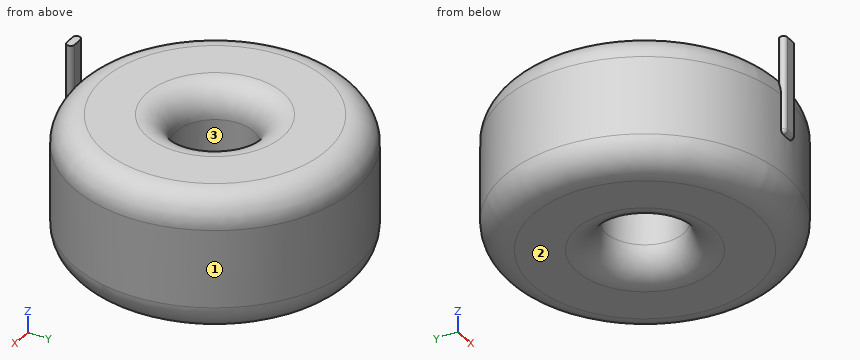
```python
from build123d import *

# Parameters (mm, degrees)
F0_R     = 72.5
F0_R_2   = 20
F1_DEPTH = 35
F2_R     = 15
F4_DEPTH = 50
F5_R     = 1.9999


# Not quite as in the source:
# - a fillet or chamfer is up to 0.001 mm smaller than in the source, because OpenCascade refuses the exact size


with BuildPart() as f1:
    # F0 (on Top) → F1 (new body, symmetric)
    with BuildSketch(Plane.XY):
        Circle(F0_R)
        Circle(F0_R_2, mode=Mode.SUBTRACT)
    extrude(amount=F1_DEPTH, both=True)

    # F2
    f2_edges = [f1.edges().sort_by_distance(p)[0] for p in [
        (-20, 0, 35),
        (20, 0, 0),
        (-20, 0, -35),
        (-72.5, 0, -35),
        (72.5, 0, 0),
        (-72.5, 0, 35),
    ]]
    fillet(f2_edges, radius=F2_R)

    # F3 (on Top) → F4 (join)
    with BuildSketch(Plane.XY):
        with BuildLine():
            Line((2.5, -70.4568837309), (-2.5, -70.4568837309))
            ThreePointArc((-2.5, -70.4568837309), (-4.5, -72.4568837309), (-2.5, -74.4568837309))
            Line((-2.5, -74.4568837309), (2.5, -74.4568837309))
            ThreePointArc((2.5, -74.4568837309), (4.5, -72.4568837309), (2.5, -70.4568837309))
        make_face()
    extrude(amount=F4_DEPTH)

    # F5 (radius 2 in the source; OpenCascade refuses exactly that, so slightly less here)
    f5_edges = [f1.edges().sort_by_distance(p)[0] for p in [
        (0, -74.456884, 0),
    ]]
    fillet(f5_edges, radius=F5_R)


solid = f1.part
```
Design review of the part built by this model. Coordinates are the model's own, in mm. Face numbers are marked on the shaded views. Give positions to 0.01 mm unless a question says otherwise; leave off trailing zeros. Loops run counter-clockwise (first coordinate to the right, second up) from the corner with the lowest first, then second, coordinate; pieces in that order, holes last. Notation, with made-up numbers: M 64,28.5 L 74,28.5 A21 ccw 74,67.5 Z; hole C 10.25,83.25 d8. An arc over 180 degrees is marked long. Return JSON: item names as keys, results as strings. Group by question number.
Item 1: For probe 1 along Y at (x, z) = (0, 9); probe 2 along Y at (x, z) = (0, -10); probe 3 along Z at (x, y) = (23, 53), list the stretches that pass through material, from the lowest coordinate up.
Item 2: We need section A-A (y = 0). Give the boundary of the cut face in (x, z).
Item 3: We need section C-C (z = -4). Give the boundary of the cut face in (x, y), and give its area (3 significant figures).
Item 4: We need section D-D (z = 7.5). Give the boundary of the cut face in (x, y), and give its area (3 significant figures).
Item 5: Insertion check: pin 1 Ø1.5 at (y, z) = (30.5, 28) entering from -X; pin 2 Ø1 at (y, z) = (30.5, -10.5) entering from -X; pin 3 Ø1 at (x, y) = (-54.5, 28.5) entering from +Z. Each pin has a flat end and moves straight along its axis. Give the tip position at first contact, or say it passes through.
Item 6: We need section B-B (z = 43.5). Give the boundary of the cut face in (x, y), and give its area (3 significant figures).
Item 7: Mouldability with a two-part tool opening along X and no side actions: class the marked faces 1, 2 and 3 as released by +X, released by -X, zero draft, split by the parting line, or undercut.
Output:
{
 "1": {"probe 1": "y = -74.46 to -20, 20 to 72.5", "probe 2": "y = -72.5 to -20, 20 to 72.5", "probe 3": "z = -35 to 35"},
 "2": {"outline": "M -72.5,-20 A15 ccw -57.5,-35 L -35,-35 A15 ccw -20,-20 L -20,20 A15 ccw -35,35 L -57.5,35 A15 ccw -72.5,20 Z; M 20,-20 A15 ccw 35,-35 L 57.5,-35 A15 ccw 72.5,-20 L 72.5,20 A15 ccw 57.5,35 L 35,35 A15 ccw 20,20 Z"},
 "3": {"outline": "C 0,0 d145; hole C 0,0 d40", "area": "15,300 mm^2"},
 "4": {"outline": "M -4.5,-72.36 A2 ccw -2.5,-74.46 L 2.5,-74.46 A2 ccw 4.5,-72.36 A72.5 ccw long Z; hole C 0,0 d40", "area": "15,300 mm^2"},
 "5": {"pin 1": "stops at x = -63.83", "pin 2": "stops at x = -66", "pin 3": "stops at z = 34.59"},
 "6": {"outline": "M -2.5,-74.46 L 2.5,-74.46 A2 ccw 2.5,-70.46 L -2.5,-70.46 A2 ccw Z", "area": "32.6 mm^2"},
 "7": {"face 1": "split by the parting line", "face 2": "zero draft", "face 3": "undercut"}
}
